Geometry check sheet. Reference: the model listing, model coordinates, mm. Face numbers are marked on the shaded views. A direction names the side the tool comes from. Coordinates: 2 decimals unless noted, no trailing zeros. Write each loop counter-clockwise with the first axis right and the second up, starting at its lowest first coordinate (ties: lowest second). Pieces come first, ordered by that corner, then holes. Notation, with made-up numbers: M 70.25,-7 L 75.25,-7 A20 cw 75.25,13 Z; hole C -28,76 d3. An arc over 180 degrees is marked long. Write item = value, one per line. Start each with the question number.
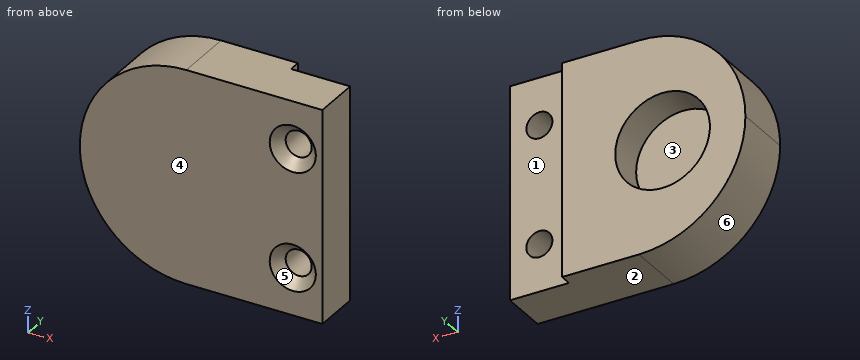
Autodesk Inventor part; units mm, degrees
ref_plane "YZ Plane" through (0, 0, 0) normal (1, 0, 0) x (0, 1, 0)
ref_plane "XZ Plane" through (0, 0, 0) normal (0, 1, 0) x (-1, 0, 0)
ref_plane "XY Plane" through (0, 0, 0) normal (0, 0, 1) x (1, 0, 0)
sketch "Эскиз1" plane through (0, 0, 0) normal (0, 1, 0) x (-1, 0, 0)
  line L0 (0, 0) -> (20.5, 0)
  line L1 (20.5, 0) -> (20.5, -18)
  line L2 (20.5, -18) -> (0, -18)
  line L3 (0, -18) -> (0, 0)
  dimension "d0" = 20.5
  dimension "d1" = 18
extrude "Выдавливание1" add sketch "Эскиз1" along normal blind 5
sketch "Эскиз2" plane through (0, 5, 0) normal (0, 1, 0) x (1, 0, 0)
  line L0 (-20.5, 18) -> (-20.5, 0)
  line L1 (-20.5, 9) -> (-13.5, 9)
  circle A0 centre (-13.5, 9) radius 4
  point P0 (0, 0)
  dimension "d4" = 7
  dimension "d5" = 8
extrude "Выдавливание2" cut sketch "Эскиз2" against normal blind 3
fillet "Сопряжение1" radius 9 2 edges at (-20.5, 2.5, 0) (-20.5, 2.5, -18)
sketch "Эскиз3" plane through (0, 0, 0) normal (0, -1, 0) x (1, 0, 0)
  line L0 (0, 0) -> (0, -18)
  line L1 (0, -9) -> (-2.5, -9)
  line L2 (-2.5, -4) -> (-2.5, -14)
  dimension "d9" = 2.5
  dimension "d10" = 10
hole "Отверстие1" at (-2.5, 0, -4) at (-2.5, 0, -14) direction (0, 1, 0) diameter 2.2 end through all countersink diameter 3.9 countersink angle 90
sketch "Эскиз4" plane through (0, 5, 0) normal (0, 1, 0) x (1, 0, 0)
  line L0 (0, 0) -> (-5, 0)
  line L1 (-5, 0) -> (-5, 18)
  line L2 (-5, 18) -> (0, 18)
  line L3 (0, 18) -> (0, 0)
  line L4 (0, 18) -> (-11.5, 18)
  dimension "d18" = 5
extrude "Выдавливание3" cut sketch "Эскиз4" against normal blind 1
properties part number "Деталь основы рулевого управления"
Q1. Gauge pin test, flat ends, axial feed: pin 1 (1.3 mm diameter, centred on x = -2.5, z = -4, fed in from -Y); pin 2 (3 mm diameter, centred on y = 1.5, z = -6, fed in from +X); pin 3 (0.8 mm diameter, centred on y = 4.5, z = -10, fed in from +X); pin 4 (1 mm diameter, centred on y = 2, z = -15.5, fed in from -X). Record the tip position at first contact, or that the pin passes through.
Q2. Cross-section at C-C on x = -13.5. Enter the section's corners in (y, z).
Q3. Set-up check for the marked faces 1, 2 and 3: record each of +Z, -Z, +X, -X, +Y, -Y from which the full face is reachable in a straight line by a thin tool's end or side.
Q4. Cross-section at A-A on y = 3.5. Count the separate pieces of the cut face and the enclosed holes in it, and give its area (3 significant figures).
Q5. Cross-section at B-B on z = -4. Enter the section's corners in (x, y), and give its area (3 significant figures).
Q6. Scan lines: L1, parallel to Z at x = -2.5, y = 3.3; L2, parallel to Z at x = -3, y = 2.9; L3, parallel to X at y = 0.6, z = -15. Record each from-to range of solid material in increasing order.
Q7. Cross-section at D-D on z = -16.25. Enter the section's corners in (x, y), and give its area (3 significant figures).
Q8. Draft check along Z on the marked faces 4, 5 and 6. Enter one of: pulls with the +Z half, pulls with the -Z half, needs draft (parallel to the pull), parting line crosses it, or undercut.
Values found:
q1.pin_1 = through
q1.pin_2 = 0
q1.pin_3 = -5
q1.pin_4 = -18.21
q2.outline = M 0,-17.78 L 5,-17.78 L 5,-13 L 2,-13 L 2,-5 L 5,-5 L 5,-0.22 L 0,-0.22 Z
q3.face_1 = +Z, -Z, +X, +Y
q3.face_2 = -Z, +X, -X, +Y, -Y
q3.face_3 = +Y
q4.separate_pieces = 1
q4.enclosed_holes = 3
q4.area = 276 mm²
q5.outline = M -18.98,0 L -4.45,0 L -3.6,0.85 L -3.6,4 L -5,4 L -5,5 L -18.98,5 Z; M -1.4,0.85 L -0.55,0 L 0,0 L 0,4 L -1.4,4 Z
q5.area = 80.4 mm²
q6.L1 = -18 to -15.1, -12.9 to -5.1, -2.9 to 0
q6.L2 = -18 to -14.98, -13.02 to -4.98, -3.02 to 0
q6.L3 = -18.21 to -3.41, -1.59 to 0
q7.outline = M -16.83,0 L 0,0 L 0,4 L -5,4 L -5,5 L -16.83,5 Z
q7.area = 79.2 mm²
q8.face_4 = needs draft
q8.face_5 = undercut
q8.face_6 = pulls with the -Z half
